Here's how the part is built. I have some questions about the finished solid (model axes, mm). Give positions to 0.01 mm unless a question says otherwise; leave off trailing zeros. Order: outer loops, then holes, each group sorted by start corner. A loop starts at its lowest first (then second) coordinate and runs counter-clockwise, first axis right, second up. Notation, with made-up numbers: M 48,-40 L 95,-40 A22 cw 95,-19 Z; hole C 29,3 d5. An arc over 180 degrees is marked long. Use one line per item in the form item = value.
from build123d import *

# Parameters (mm, degrees)
SKETCH1_W                      = 220
SKETCH1_H                      = 158
BOSS_EXTRUDE1_DEPTH            = 5.5
CBORE_FOR_M4_SHCS1_D           = 4.5
CBORE_FOR_M4_SHCS1_CBORE_D     = 8
CBORE_FOR_M4_SHCS1_CBORE_DEPTH = 4
SKETCH6_W                      = 20
SKETCH6_H                      = 40
CUT_EXTRUDE2_DEPTH             = 6.5


with BuildPart() as part:
    # Sketch1 → Boss-Extrude1 (new body)
    with BuildSketch(Plane(origin=(0, 0, 0), x_dir=(1, 0, 0), z_dir=(0, 1, 0))):
        Rectangle(SKETCH1_W, SKETCH1_H)
    extrude(amount=BOSS_EXTRUDE1_DEPTH)

    # CBORE for M4 SHCS1 (through all)
    with Locations(Plane.XZ):
        with Locations((100, 0)):
            cbore_for_m4_shcs1 = CounterBoreHole(CBORE_FOR_M4_SHCS1_D / 2, CBORE_FOR_M4_SHCS1_CBORE_D / 2, CBORE_FOR_M4_SHCS1_CBORE_DEPTH)

    # Mirror2: CBORE for M4 SHCS1 across plane
    add(cbore_for_m4_shcs1.mirror(Plane(origin=(0, 0, 0), x_dir=(0, 0, 1), z_dir=(1, 0, 0))), mode=Mode.SUBTRACT)

    # Sketch6 → Cut-Extrude2 (cut, through all)
    with BuildSketch(Plane(origin=(0, 5.5, 0), x_dir=(1, 0, 0), z_dir=(0, 1, 0))):
        with Locations((100, 59)):
            Rectangle(SKETCH6_W, SKETCH6_H)
    cut_extrude2 = extrude(amount=-CUT_EXTRUDE2_DEPTH, mode=Mode.SUBTRACT)

    # Mirror3: Cut-Extrude2 across plane
    add(cut_extrude2.mirror(Plane.XY), mode=Mode.SUBTRACT)


solid = part.part
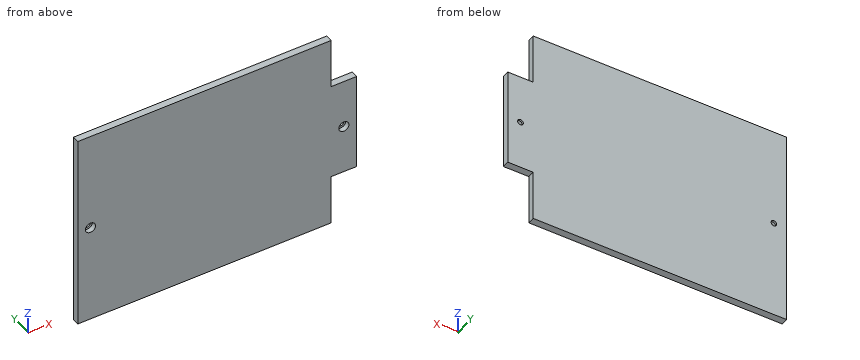
Q1. I'm going to push flat-ended pins straight in: pin 1 Ø2.5 at (x, z) = (99, 2) entering from -Y; pin 2 Ø3 at (y, z) = (2.5, -65.5) entering from +X; pin 3 Ø9 at (x, z) = (100, 0) entering from +Y; pin 4 Ø3 at (x, y) = (102.5, 2.5) entering from -Z. Where does each tip first touch, or does it pass through?
Found:
pin_1 = 4
pin_2 = 90
pin_3 = 5.5
pin_4 = -39
Q2. I want a section at A-A on x = -100. Write out the boundary of the cut face in (y, z).
Found:
outline = M 0,-79 L 5.5,-79 L 5.5,-2.25 L 4,-2.25 L 4,-4 L 0,-4 Z; M 0,4 L 4,4 L 4,2.25 L 5.5,2.25 L 5.5,79 L 0,79 Z
Q3. I want a section at B-B on z = 0. Write out the boundary of the cut face in (x, y), then the cut area to 3 significant figures.
Found:
outline = M -110,0 L -104,0 L -104,4 L -102.25,4 L -102.25,5.5 L -110,5.5 Z; M -97.75,4 L -96,4 L -96,0 L 96,0 L 96,4 L 97.75,4 L 97.75,5.5 L -97.75,5.5 Z; M 102.25,4 L 104,4 L 104,0 L 110,0 L 110,5.5 L 102.25,5.5 Z
area = 1,130 mm²
Q4. I want a section at D-D on x = 100. Write out the boundary of the cut face in (y, z).
Found:
outline = M 0,-39 L 5.5,-39 L 5.5,-2.25 L 4,-2.25 L 4,-4 L 0,-4 Z; M 0,4 L 4,4 L 4,2.25 L 5.5,2.25 L 5.5,39 L 0,39 Z
Q5. I need wall thicknesses on L1, parallel to Z at x = 100, y = 4.45; L2, parallel to Z at x = -99.5, y = 2.1; L3, parallel to X at y = 4.75, z = 0.5. Which ranges of each line are inside material? Lowest first, please.
Found:
L1 = -39 to -2.25, 2.25 to 39
L2 = -79 to -3.97, 3.97 to 79
L3 = -110 to -102.19, -97.81 to 97.81, 102.19 to 110
Q6. I want a section at C-C on y = 3.05. Write out the boundary of the cut face in (x, z), then the cut area to 3 significant figures.
Found:
outline = M -110,-79 L 90,-79 L 90,-39 L 110,-39 L 110,39 L 90,39 L 90,79 L -110,79 Z; hole C -100,0 d8; hole C 100,0 d8
area = 33,100 mm²
